Design review of the part built by this model. Coordinates are the model's own, in mm. A direction names the side the tool comes from. Coordinates: 2 decimals unless noted, no trailing zeros. Write each loop counter-clockwise with the first axis right and the second up, starting at its lowest first coordinate (ties: lowest second). Pieces come first, ordered by that corner, then holes. Notation, with made-up numbers: M -13,-2 L 18,-2 A26 ccw 18,14 Z; hole C -38.5,77 d11. An arc over 180 degrees is marked long. Write item = value, one per line.
Autodesk Inventor part; units mm, degrees
ref_plane "Work Plane1" through (-56.3599, 0, 22) normal (0, 0, -1) x (-1, 0, 0)
ref_plane "YZ Plane" through (0, 0, 0) normal (1, 0, 0) x (0, 1, 0)
ref_plane "XZ Plane" through (0, 0, 0) normal (0, 1, 0) x (-1, 0, 0)
ref_plane "Work Plane1" through (-56.3599, 0, 22) normal (0, 0, -1) x (-1, 0, 0)
sketch "Sketch1" plane through (-56.3599, 0, 22) normal (0, 0, -1) x (-1, 0, 0)
  line L0 (-4.0299, -0.3538) -> (-2.2322, 1.4439) construction
  arc A0 (-1.4439, 2.2322) -> (-2.2322, 1.4439) centre (-0.9299, 0.9299) ccw construction
  line L1 (-1.4439, 2.2322) -> (0.3538, 4.0299) construction
  line L2 (-37.8299, 42.8299) -> (-37.8299, 37.8299) construction
  line L3 (-37.8299, 37.8299) -> (-42.9208, 37.8299) construction
  line L4 (-37.8299, 42.2137) -> (-37.8299, 45.8299) construction
  line L5 (-37.8299, 45.8299) -> (-4.0299, 45.8299) construction
  line L6 (-4.0299, 45.8299) -> (-4.0299, 42.2137) construction
  line L7 (-4.0299, 4.0299) -> (0.3538, 4.0299)
  circle A1 centre (-20.9299, 20.9299) radius 17.5
  line L8 (-20.9299, 58.9723) -> (17.1124, 20.9299) construction
  line L9 (17.1124, 20.9299) -> (-20.9299, -17.1124) construction
  line L10 (-20.9299, -17.1124) -> (-58.9723, 20.9299) construction
  line L11 (-58.9723, 20.9299) -> (-20.9299, 58.9723) construction
  line L12 (-20.9299, 58.9723) -> (-20.9299, -17.1124) construction
  line L13 (17.1124, 20.9299) -> (-58.9723, 20.9299) construction
  line L14 (-20.9299, 58.9723) -> (32.8701, 58.9723) construction
  line L15 (-43.4299, 43.4299) -> (1.5701, 43.4299) construction
  line L16 (1.5701, 43.4299) -> (1.5701, -1.5701) construction
  line L17 (1.5701, -1.5701) -> (-43.4299, -1.5701) construction
  line L18 (-43.4299, -1.5701) -> (-43.4299, 43.4299) construction
  line L19 (-43.4299, 43.4299) -> (1.5701, -1.5701) construction
  line L20 (1.5701, 43.4299) -> (-43.4299, -1.5701) construction
  line L21 (-43.4299, 5.3876) -> (-43.4299, 36.4723)
  line L22 (-43.4299, 36.4723) -> (-36.4723, 43.4299)
  line L23 (-36.4723, 43.4299) -> (-5.3876, 43.4299)
  line L24 (-5.3876, 43.4299) -> (1.5701, 36.4723)
  line L25 (1.5701, 36.4723) -> (1.5701, 5.3876)
  line L26 (1.5701, 5.3876) -> (-5.3876, -1.5701)
  line L27 (-5.3876, -1.5701) -> (-36.4723, -1.5701)
  line L28 (-36.4723, -1.5701) -> (-43.4299, 5.3876)
  line L29 (-4.0299, 42.2137) -> (-37.8299, 42.2137)
  line L30 (-4.0299, -0.3538) -> (-4.0299, 4.0299)
  circle A2 centre (-20.9299, 20.9299) radius 1.5
  line L31 (-10.9299, 10.9299) -> (-30.9299, 10.9299) construction
  line L32 (-30.9299, 10.9299) -> (-30.9299, 30.9299) construction
  line L33 (-30.9299, 30.9299) -> (-10.9299, 30.9299) construction
  line L34 (-10.9299, 30.9299) -> (-10.9299, 10.9299) construction
  line L35 (-10.9299, 10.9299) -> (-30.9299, 30.9299) construction
  line L36 (-30.9299, 10.9299) -> (-10.9299, 30.9299) construction
  circle A3 centre (-30.9299, 30.9299) radius 1.4
  circle A4 centre (-30.9299, 10.9299) radius 1.4
  circle A5 centre (-10.9299, 10.9299) radius 1.4
  line L37 (-45.8299, 37.8299) -> (-42.0723, 37.8299) construction
  line L38 (-42.1723, 37.7299) -> (-45.8299, 37.7299)
  line L39 (-45.8299, 37.7299) -> (-45.8299, 4.1299)
  line L40 (-45.8299, 4.1299) -> (-42.1723, 4.1299)
  line L41 (-42.1723, 4.1299) -> (-42.1723, 37.7299)
  line L42 (-45.8299, 4.0299) -> (-42.0723, 4.0299) construction
  line L43 (-45.8299, 37.8299) -> (-42.0723, 37.8299)
  line L44 (-37.7299, 45.8299) -> (-4.1299, 45.8299)
  line L45 (-4.1299, 45.8299) -> (-4.1299, 42.1723)
  line L46 (-4.1299, 42.1723) -> (-37.7299, 42.1723)
  line L47 (-37.7299, 42.1723) -> (-37.7299, 45.8299)
  line L48 (0.4701, 37.8299) -> (0.4701, 4.0299) construction
  line L49 (0.4701, 4.0299) -> (3.9701, 4.0299) construction
  line L50 (3.9701, 37.8299) -> (3.9701, 4.0299) construction
  line L51 (0.4701, 37.8299) -> (3.9701, 37.8299) construction
  line L52 (-45.8299, -3.9701) -> (-4.0299, -3.9701) construction
  line L53 (0.3124, 37.7299) -> (3.9701, 37.7299)
  line L54 (3.9701, 37.7299) -> (3.9701, 4.1299)
  line L55 (3.9701, 4.1299) -> (0.3124, 4.1299)
  line L56 (0.3124, 4.1299) -> (0.3124, 37.7299)
  line L57 (-4.1713, -0.3538) -> (-37.7299, -0.3538)
  line L58 (-37.7299, -0.3538) -> (-37.7299, -3.9701)
  line L59 (-37.7299, -3.9701) -> (-4.1713, -3.9701)
  line L60 (-4.1713, -3.9701) -> (-4.1713, -0.3538)
  point P0 (-37.8299, 4.0299)
  dimension "d18" = 53.8
  dimension "d19" = 45
  dimension "d20" = 53.8
  dimension "d21" = 45
  dimension "d22" = 45
  dimension "d30" = 20
  dimension "d31" = 20
  dimension "d32" = 2.8
  dimension "d33" = 2.8
  dimension "d34" = 2.8
  dimension "d35" = 3
  dimension "d36" = 0.1
  dimension "d37" = 0.1
  dimension "d38" = 0.1
  dimension "d39" = 0.1
extrude "Extrusion1" add sketch "Sketch1" along normal blind 12 contours L30 L26 L57 L28 L41 L22 L46 L24 L56 L7 | L7 L26 L30 | L56 L24 L25 L26 | L26 L25 L24 L53 L54 L55 | L60 L59 L58 L57 L28 L27 L26 | L26 L27 L28 L57 | L46 L22 L29 L24 | L24 L29 L45 | L40 L39 L38 L22 L21 L28 | L28 L21 L22 L41 | L29 L22 L23 L24 | L24 L23 L22 L29 L47 L44 L45 | L47 L29 L22 | A1 | A2 | A3 | A4 | A5
sketch "Skizze4" plane through (-56.3599, 0, 10) normal (0, 0, -1) x (-1, 0, 0)
  line L0 (-37.7299, 42.1723) -> (-42.1723, 37.7299)
  line L1 (-42.1723, 37.7299) -> (-45.8299, 37.7299)
  line L2 (-45.8299, 37.7299) -> (-45.8299, 4.1299) construction
  line L3 (-45.8299, 4.1299) -> (-42.1723, 4.1299)
  line L4 (-42.1723, 4.1299) -> (-37.6885, -0.3538)
  line L5 (-37.6885, -0.3538) -> (-37.7299, -0.3538)
  line L6 (-37.7299, -0.3538) -> (-37.7299, -3.9701)
  line L7 (-37.7299, -3.9701) -> (-4.1713, -3.9701) construction
  line L8 (-4.1713, -3.9701) -> (-4.1713, -0.3538)
  line L9 (-4.1713, -0.3538) -> (0.3124, 4.1299)
  line L10 (0.3124, 4.1299) -> (3.9701, 4.1299)
  line L11 (3.9701, 4.1299) -> (3.9701, 37.7299) construction
  line L12 (3.9701, 37.7299) -> (0.3124, 37.7299)
  line L13 (0.3124, 37.7299) -> (-4.1299, 42.1723)
  line L14 (-4.1299, 42.1723) -> (-4.1299, 45.8299)
  line L15 (-4.1299, 45.8299) -> (-37.7299, 45.8299) construction
  line L16 (-37.7299, 45.8299) -> (-37.7299, 42.1723)
  line L17 (-37.9299, 46.0299) -> (-3.9299, 46.0299) construction
  line L18 (-3.9299, 46.0299) -> (-3.9299, 42.2551)
  line L19 (-3.9299, 42.2551) -> (0.3953, 37.9299)
  line L20 (0.3953, 37.9299) -> (4.1701, 37.9299)
  line L21 (4.1701, 37.9299) -> (4.1701, 3.9299) construction
  line L22 (4.1701, 3.9299) -> (0.3953, 3.9299)
  line L23 (0.3953, 3.9299) -> (-3.9713, -0.4367)
  line L24 (-3.9713, -0.4367) -> (-3.9713, -4.1701)
  line L25 (-3.9713, -4.1701) -> (-37.9299, -4.1701) construction
  line L26 (-37.9299, -4.1701) -> (-37.9299, -0.3953)
  line L27 (-37.9299, -0.3953) -> (-42.2551, 3.9299)
  line L28 (-42.2551, 3.9299) -> (-46.0299, 3.9299)
  line L29 (-46.0299, 3.9299) -> (-46.0299, 37.9299) construction
  line L30 (-46.0299, 37.9299) -> (-42.2551, 37.9299)
  line L31 (-42.2551, 37.9299) -> (-37.9299, 42.2551)
  line L32 (-37.9299, 42.2551) -> (-37.9299, 46.0299)
  line L33 (-45.8299, 37.7299) -> (-45.8299, 37.9299)
  line L34 (-4.1299, 45.8299) -> (-37.7299, 45.8299)
  line L35 (-37.7299, 45.8299) -> (-37.9299, 45.8299)
  line L36 (-4.1299, 45.8299) -> (-3.9299, 45.8299)
  line L37 (3.9701, 37.7299) -> (3.9701, 37.9299)
  line L38 (3.9701, 4.1299) -> (3.9701, 37.7299)
  line L39 (3.9701, 4.1299) -> (3.9701, 3.9299)
  line L40 (-4.1713, -3.9701) -> (-3.9713, -3.9701)
  line L41 (-37.7299, -3.9701) -> (-37.9299, -3.9701)
  line L42 (-45.8299, 4.1299) -> (-45.8299, 3.9299)
  point P0 (-56.3599, 0)
  dimension "d40" = 0.2
extrude "IM_offset" add sketch "Skizze4" against normal up to surface (12 mm away)
ref_plane "Arbeitsebene5" through (-35.4299, 3.9299, 22) normal (-1, 0, 0) x (0, 0, 1)
ref_plane "Arbeitsebene6" through (-18.4299, 20.9299, 22) normal (0, 1, 0) x (-1, 0, 0)
sketch "Skizze31" plane through (-56.3599, 0, 10) normal (0, 0, -1) x (-1, 0, 0)
  line L0 (3.9701, 3.9299) -> (3.9701, 37.9299)
  line L1 (3.9701, 37.9299) -> (0.3953, 37.9299)
  line L2 (0.3953, 37.9299) -> (-3.9299, 42.2551)
  line L3 (-3.9299, 42.2551) -> (-3.9299, 45.8299)
  line L4 (-3.9299, 45.8299) -> (-37.9299, 45.8299)
  line L5 (-37.9299, 45.8299) -> (-37.9299, 42.2551)
  line L6 (-37.9299, 42.2551) -> (-42.2551, 37.9299)
  line L7 (-42.2551, 37.9299) -> (-45.8299, 37.9299)
  line L8 (-45.8299, 37.9299) -> (-45.8299, 3.9299)
  line L9 (-42.2551, 3.9299) -> (-45.8299, 3.9299)
  line L10 (-37.9299, -0.3953) -> (-42.2551, 3.9299)
  line L11 (-37.9299, -3.9701) -> (-37.9299, -0.3953)
  line L12 (-3.9713, -3.9701) -> (-37.9299, -3.9701)
  line L13 (-3.9713, -3.9701) -> (-3.9713, -0.4367)
  line L14 (-3.9713, -0.4367) -> (0.3953, 3.9299)
  line L15 (0.3953, 3.9299) -> (3.9701, 3.9299)
  line L16 (-11.9299, 27.4299) -> (-27.4299, 27.4299)
  line L17 (-11.9299, 14.4299) -> (-11.9299, 27.4299)
  line L18 (-27.4299, 14.4299) -> (-11.9299, 14.4299)
  line L19 (-27.4299, 27.4299) -> (-27.4299, 14.4299)
  circle A0 centre (-20.9299, 20.9299) radius 4.5
  circle A1 centre (-25.6799, 25.6799) radius 0.75
  circle A2 centre (-25.6799, 16.1799) radius 0.75
  circle A3 centre (-16.1799, 16.1799) radius 0.75
  circle A4 centre (-16.1799, 25.6799) radius 0.75
  line L20 (-27.6299, 14.2299) -> (-11.7299, 14.2299)
  line L21 (-11.7299, 14.2299) -> (-11.7299, 27.6299)
  line L22 (-11.7299, 27.6299) -> (-27.6299, 27.6299)
  line L23 (-27.6299, 27.6299) -> (-27.6299, 14.2299)
  point P0 (-56.3599, 0)
  dimension "d184" = 0.2
extrude "Extrusion26" cut sketch "Skizze31" against normal blind 10 contours L17 L18 L19 L16 | A0 | A1 | A2 | A3 | A4 | L23 L22 L21 L20
sketch "Skizze32" plane through (-56.3599, 0, 22) normal (0, 0, 1) x (1, 0, 0)
  circle A0 centre (20.9299, 20.9299) radius 4.5
  circle A1 centre (25.6799, 25.6799) radius 1.25
  circle A2 centre (16.1799, 16.1799) radius 1.25
  circle A3 centre (25.6799, 16.1799) radius 1.25
  circle A4 centre (16.1799, 25.6799) radius 1.25
  line L0 (14.4299, 27.4299) -> (27.4299, 27.4299)
  line L1 (27.4299, 27.4299) -> (27.4299, 14.4299)
  line L2 (27.4299, 14.4299) -> (14.4299, 14.4299)
  line L3 (14.4299, 14.4299) -> (14.4299, 27.4299)
  circle A5 centre (16.1799, 25.6799) radius 1.25
  circle A6 centre (16.1799, 25.6799) radius 1.5
  circle A7 centre (25.6799, 25.6799) radius 1.5
  circle A8 centre (25.6799, 16.1799) radius 1.5
  circle A9 centre (16.1799, 16.1799) radius 1.5
  point P0 (56.3599, 0)
  dimension "d187" = 13
  dimension "d188" = 13
  dimension "d189" = 9
  dimension "d190" = 2.5
  dimension "d191" = 1.75
  dimension "d192" = 9.5
  dimension "d193" = 1.75
  dimension "d194" = 3
  dimension "d195" = 3
  dimension "d196" = 3
  dimension "d197" = 3
extrude "Extrusion27" cut sketch "Skizze32" against normal blind 10 contours A0 | A1 | A2 | A3 | A4 | A6 | A7 | A8 | A9
properties part number "20_Cube_Insert_Lasertack_mount_v3"
Q1. Wall thickness on line 1 (Y direction, x = -30.68, z = 21.55); line 2 (Y direction, x = -36.5, z = 15.75); line 3 (X direction, y = 43, z = 11): over which ranges is each line inside the solid? List them lowest first.
Check result:
line_1 = -3.97 to 14.68, 17.68 to 24.18, 27.18 to 45.83
line_2 = -3.97 to 14.23, 27.63 to 45.83
line_3 = -52.43 to -18.43
Q2. Consider section C-C, the plane y = 20. State the section outline as (x, z) points.
Check result:
outline = M -60.33,10 L -44.63,10 L -44.63,20 L -39.83,20 L -39.83,22 L -60.33,22 Z; M -31.03,20 L -28.73,20 L -28.73,10 L -10.53,10 L -10.53,22 L -31.03,22 Z
Q3. For P1, Ø1.1, axis at x = -58.5, z = 15, coming from the +Y side; P2, Ø3, axis at y = 44.5, z = 17, coming from the -X side; P3, Ø4, axis at x = -13, z = 15.5, coming from the +Y side, all flat-tipped, find the tip position at first contact; note any pin that passes through.
Check result:
P1 = 37.93
P2 = -52.43
P3 = 38.83
Q4. Machinability: for faces 4 (the flat face through (-18.43, -2, 16)), 5 (the flat face through (-37, 14.23, 15)), 6 (the flat face through (-59, 3.93, 16)), which of the approach directions +Z, -Z, +X, -X, +Y, -Y give a long, thin tool a straight path to every point of the face, cutting with its end or side? Answer none if there is none.
Check result:
face_4 = +Z, -Z, +X, -Y
face_5 = -Z
face_6 = +Z, -Z, -X, -Y
Q5. Consider section A-A, the plane x = -35.43. State the section outline as (y, z) points, and give its area (3 significant figures).
Check result:
outline = M -3.97,10 L 14.23,10 L 14.23,20 L 16.43,20 L 16.43,22 L -3.97,22 Z; M 25.43,20 L 27.63,20 L 27.63,10 L 45.83,10 L 45.83,22 L 25.43,22 Z
area = 446 mm²
Q6. The part is to be moulded in two halves that separate along X. For faces 1 (the flat face through (-35, 45.83, 16)), 2 (the flat face through (-40.1, 21, 20)), 3 (the flat face through (-16.298, 1.737, 15.916)), say which applies: +X half, -X half, draft (parallel to the pull), parting line (faces both ways), or undercut.
Check result:
face_1 = draft
face_2 = undercut
face_3 = +X half
Q7. Consider section B-B, the plane z = 18.75. State the section outline as (x, y) points.
Check result:
outline = M -60.33,3.93 L -56.76,3.93 L -52.39,-0.44 L -52.39,-3.97 L -18.43,-3.97 L -18.43,-0.4 L -14.1,3.93 L -10.53,3.93 L -10.53,37.93 L -14.1,37.93 L -18.43,42.26 L -18.43,45.83 L -52.43,45.83 L -52.43,42.26 L -56.76,37.93 L -60.33,37.93 Z; hole M -44.63,14.23 L -28.73,14.23 L -28.73,27.63 L -44.63,27.63 Z
